Model file for the job. Use its own axes, mm. A direction names the side the tool comes from. Round coordinates to 2 decimals unless told otherwise and drop trailing zeros. Loops run counter-clockwise (first coordinate to the right, second up) from the corner with the lowest first, then second, coordinate; pieces in that order, holes last. Notation, with made-up numbers: M 31,72 L 70,72 A25 ccw 70,104 Z; hole C -38.5,13.5 d10. An arc over 180 degrees is marked long. Use a Markdown table: item, result. Add a question column.
Q1. Cut at B-B (x = 49). Give the cut face in (y, z), plus the area to 3 significant figures.
Q2. Pin check, flat tips, straight feed: pin 1 (0.5 mm diameter, centred on y = 3, z = 1.5, fed in from -X); pin 2 (0.6 mm diameter, centred on x = 28, z = 1, fed in from -Y); pin 3 (1.5 mm diameter, centred on x = 37.5, z = 1.5, fed in from -Y). Stop position of each tip, or through.
Q3. Probe line 1 (X direction, y = 0.75, z = 0.9); line 2 (X direction, y = -1.5, z = 0.6); line 3 (X direction, y = -3, z = 1.1). List the from-to ranges inside material, lowest first. Write a range as from..to.
Q4. Tool access for faces 1 (the face through (9, -4, 3)), 2 (the face through (54.999, -10, 2)), 3 (the face through (16, -2.907, 2)): list every direction of +Z, -Z, +X, -X, +Y, -Y with a clear straight run to the whole face (end or side of a thin tool).
Q5. Cut at D-D (z = 1.25). State how many separate pieces and enclosed holes the cut face has, plus the area to 3 significant figures.
Q6. Cut at C-C (y = 5). Give the cut face in (x, z), plus the area to 3 significant figures.
Q7. Cut at A-A (y = 10.25). Give the cut face in (x, z).
Q8. Mould opens along Y. For faces 4 (the face through (0, -5, 2)), 5 (the face through (47, -8.416, 2)), 6 (the face through (36, -4.416, 2)) say: +Y half, -Y half, draft (parallel to the pull), parting line (faces both ways), or undercut.
from build123d import *

# Parameters (mm, degrees)
SKETCH_1_W          = 2.3276
SKETCH_1_H          = 1.694
EXTRUDE_1_DEPTH     = 3
CUT_EXTRUDE_1_DEPTH = 1


with BuildPart() as part:
    # 草图1 → 凸台-拉伸1 (new body)
    with BuildSketch(Plane.XY.offset(3)):
        with BuildLine():
            Line((23.2531, 5.583631793), (24.503, 5.583631793))
            Line((24.503, 5.583631793), (24.503, 9.583631793))
            Line((24.503, 9.583631793), (18.3721, 9.583631793))
            Line((18.3721, 9.583631793), (18.3721, 12.583631793))
            Line((18.3721, 12.583631793), (12.9991, 12.583631793))
            Line((12.9991, 12.583631793), (12.9991, 7.316491962))
            ThreePointArc((12.9991, 7.316491962), (11.277392164, 3.159921553), (7.120821755, 1.438213717))
            Line((7.120821755, 1.438213717), (0, 1.438213717))
            Line((0, 1.438213717), (0, -11.416368207))
            Line((0, -11.416368207), (7.4994, -11.416368207))
            Line((7.4994, -11.416368207), (7.4994, -8.416368207))
            Line((7.4994, -8.416368207), (36.5002, -8.416368207))
            Line((36.5002, -8.416368207), (36.5002, -4.416368207))
            Line((36.5002, -4.416368207), (35.2489, -4.416368207))
            Line((35.2489, -4.416368207), (35.2489, -1.916368207))
            Line((35.2489, -1.916368207), (36.5002, -1.916368207))
            Line((36.5002, -1.916368207), (36.5002, 1.583631793))
            Line((36.5002, 1.583631793), (39.5003, 1.583631793))
            Line((39.5003, 1.583631793), (39.5003, -1.916368207))
            Line((39.5003, -1.916368207), (40.7501, -1.916368207))
            Line((40.7501, -1.916368207), (40.7501, -4.416368207))
            Line((40.7501, -4.416368207), (39.5003, -4.416368207))
            Line((39.5003, -4.416368207), (39.5003, -8.416368207))
            Line((39.5003, -8.416368207), (54.9988, -8.416368207))
            Line((54.9988, -8.416368207), (54.9988, -11.416368207))
            Line((54.9988, -11.416368207), (59.9998, -11.416368207))
            Line((59.9998, -11.416368207), (59.9998, 12.583631793))
            Line((59.9998, 12.583631793), (51.9988, 12.583631793))
            Line((51.9988, 12.583631793), (51.9988, 9.583631793))
            Line((51.9988, 9.583631793), (27.5031, 9.583631793))
            Line((27.5031, 9.583631793), (27.5031, 5.583631793))
            Line((27.5031, 5.583631793), (28.7543, 5.583631793))
            Line((28.7543, 5.583631793), (28.7543, 3.083631793))
            Line((28.7543, 3.083631793), (27.5031, 3.083631793))
            Line((27.5031, 3.083631793), (27.5031, -0.416368207))
            Line((27.5031, -0.416368207), (24.503, -0.416368207))
            Line((24.503, -0.416368207), (24.503, 3.083631793))
            Line((24.503, 3.083631793), (23.2531, 3.083631793))
            Line((23.2531, 3.083631793), (23.2531, 5.583631793))
        make_face()
        with BuildLine():
            Line((46.2504, 6.082631793), (54.9998, 6.082631793))
            ThreePointArc((54.9998, 6.082631793), (56.414013562, 5.496845355), (56.9998, 4.082631793))
            Line((56.9998, 4.082631793), (56.9998, -2.916368207))
            ThreePointArc((56.9998, -2.916368207), (56.414013562, -4.330581769), (54.9998, -4.916368207))
            Line((54.9998, -4.916368207), (46.2504, -4.916368207))
            ThreePointArc((46.2504, -4.916368207), (44.836186438, -4.330581769), (44.2504, -2.916368207))
            Line((44.2504, -2.916368207), (44.2504, 4.082631793))
            ThreePointArc((44.2504, 4.082631793), (44.836186438, 5.496845355), (46.2504, 6.082631793))
        make_face(mode=Mode.SUBTRACT)
        with Locations((15.811, 3.177631793)):
            Rectangle(SKETCH_1_W, SKETCH_1_H, mode=Mode.SUBTRACT)
        with Locations((15.7586, -2.060368207)):
            Rectangle(SKETCH_1_W, SKETCH_1_H, mode=Mode.SUBTRACT)
    extrude(amount=-EXTRUDE_1_DEPTH)

    # 草图2 → 切除-拉伸1 (cut)
    # profile 1 of 2: a face of its own
    with BuildSketch(Plane.XY.offset(3)):
        Polygon((5.418488838, -1.146310398), (6.065624255, -1.146310398), (6.065624255, -4.646310398), (5.75152169, -4.646310398), (5.75152169, -1.505284757), (5.213060152, -1.505284757), align=None)
    # profile 2 of 2: a face of its own
    with BuildSketch(Plane.XY.offset(3)):
        with BuildLine():
            Line((8.982290921, -1.056566809), (9.22417794, -1.246570815))
            Line((9.22417794, -1.246570815), (8.299398293, -2.660733475))
            add(Edge.make_bspline(
                [(8.299398293, -2.660733475), (8.36096857, -2.650919615), (8.481068357, -2.63177657), (8.602634255, -2.628618624), (8.661878261, -2.627079629)],
                knots=[0, 0, 0, 0, 1.025318673, 2, 2, 2, 2], degree=3))
            add(Edge.make_bspline(
                [(8.661878261, -2.627079629), (8.697450757, -2.628035741), (8.767474158, -2.629917818), (8.87028096, -2.644401669), (8.969069896, -2.667226781), (9.063431508, -2.700499037), (9.15370449, -2.743001391), (9.240406886, -2.793940261), (9.321908896, -2.855945942), (9.399260075, -2.925210897), (9.469487173, -3.001927882), (9.531663228, -3.083329219), (9.58389002, -3.1693301), (9.626263942, -3.259886966), (9.65916882, -3.354860225), (9.683156465, -3.454128365), (9.697336058, -3.557759836), (9.699261549, -3.628238011), (9.700239639, -3.664038764)],
                knots=[0, 0, 0, 0, 1.04369286, 2.054478336, 3.041073146, 4.015093852, 4.984733326, 5.965804835, 6.960378782, 7.985147595, 9.009457201, 10.008161701, 10.986880575, 11.956520048, 12.937015923, 13.931873656, 14.949455224, 16, 16, 16, 16], degree=3))
            add(Edge.make_bspline(
                [(9.700239639, -3.664038764), (9.698816534, -3.713018468), (9.696016201, -3.809398934), (9.668112405, -3.94977564), (9.62475276, -4.083508155), (9.562775231, -4.208461327), (9.485792849, -4.324463896), (9.391915256, -4.427249362), (9.284471767, -4.518919399), (9.162984969, -4.595576018), (9.032242005, -4.658179069), (8.894890008, -4.703144311), (8.752262861, -4.730827781), (8.655458253, -4.734298384), (8.606489639, -4.736053988)],
                knots=[0, 0, 0, 0, 1.031375318, 2.029502543, 3.004789286, 3.987476834, 4.960371455, 5.9300674, 6.912260825, 7.929083631, 8.949397511, 9.960523116, 10.96833055, 12, 12, 12, 12], degree=3))
            add(Edge.make_bspline(
                [(8.606489639, -4.736053988), (8.559392939, -4.734525782), (8.466102621, -4.731498674), (8.328869826, -4.704532736), (8.197006809, -4.660825634), (8.071437428, -4.600611355), (7.955116815, -4.524553472), (7.851051179, -4.432991193), (7.759759404, -4.327881728), (7.683784783, -4.209241381), (7.623526051, -4.081751423), (7.578336126, -3.948814267), (7.551939883, -3.810914285), (7.548251326, -3.717433146), (7.546393485, -3.67034886)],
                knots=[0, 0, 0, 0, 1.012016664, 2.004627821, 2.994792927, 3.992885782, 4.990978636, 5.973936114, 6.964471063, 7.975201453, 8.993600317, 9.990122807, 10.98767138, 12, 12, 12, 12], degree=3))
            add(Edge.make_bspline(
                [(7.546393485, -3.67034886), (7.54757493, -3.634304277), (7.549987215, -3.560708125), (7.566830606, -3.449244097), (7.5938954, -3.335193015), (7.624205647, -3.238438821), (7.656231257, -3.159177299), (7.682883796, -3.095273809), (7.716057792, -3.029512736), (7.751431174, -2.9596391), (7.792188043, -2.887453667), (7.836503692, -2.811749997), (7.885603343, -2.73373207), (7.920023506, -2.680787874), (7.937619447, -2.653722257)],
                knots=[0, 0, 0, 0, 1.173818275, 2.396712641, 3.66331629, 4.989737886, 5.693666774, 6.447286557, 7.243889047, 8.091586357, 8.998013824, 9.943181721, 10.948533338, 12, 12, 12, 12], degree=3))
            Line((7.937619447, -2.653722257), (8.982290921, -1.056566809))
        make_face()
        with BuildLine():
            add(Edge.make_bspline(
                [(8.595972812, -2.986053988), (8.569310567, -2.986832032), (8.517231458, -2.988351777), (8.440824043, -2.997177029), (8.368510792, -3.013796095), (8.299333658, -3.034962426), (8.234585955, -3.064065486), (8.173797115, -3.099417285), (8.116732064, -3.141038463), (8.063988512, -3.188339374), (8.016168848, -3.240127407), (7.974987718, -3.29559693), (7.939465318, -3.353411133), (7.910583499, -3.414053075), (7.888093423, -3.477499574), (7.871825172, -3.543458824), (7.862771421, -3.61237313), (7.861265189, -3.659105633), (7.860496049, -3.682969052)],
                knots=[0, 0, 0, 0, 1.129588631, 2.206414736, 3.251139165, 4.268635594, 5.265702196, 6.250456724, 7.242448911, 8.251968645, 9.246821453, 10.222880186, 11.173611482, 12.116736599, 13.062300278, 14.020270554, 14.989073742, 16, 16, 16, 16], degree=3))
            add(Edge.make_bspline(
                [(7.860496049, -3.682969052), (7.861122411, -3.706619032), (7.862350613, -3.752993122), (7.873502932, -3.821332301), (7.890538015, -3.88709721), (7.915878411, -3.949948808), (7.946105299, -4.010845127), (7.986010623, -4.067580412), (8.030227409, -4.123600482), (8.083081342, -4.174601954), (8.139804705, -4.222058578), (8.200405908, -4.263538831), (8.263565868, -4.299025005), (8.33013729, -4.326836102), (8.399175674, -4.349660389), (8.471256228, -4.365721868), (8.546429083, -4.374802394), (8.597351021, -4.376310588), (8.623316562, -4.377079629)],
                knots=[0, 0, 0, 0, 0.989467248, 1.94019797, 2.891935182, 3.827694429, 4.772920941, 5.730924762, 6.725747692, 7.756678648, 8.79901574, 9.819492441, 10.826891316, 11.826466727, 12.835195252, 13.867842842, 14.912794438, 16, 16, 16, 16], degree=3))
            add(Edge.make_bspline(
                [(8.623316562, -4.377079629), (8.649282061, -4.376310528), (8.700203915, -4.374802216), (8.775377376, -4.365722547), (8.847455694, -4.349657899), (8.916502203, -4.326845129), (8.983043634, -4.298991519), (9.046148355, -4.263759599), (9.106176449, -4.221803482), (9.162937048, -4.174683053), (9.215570987, -4.123310201), (9.260848266, -4.068080479), (9.299531499, -4.010386584), (9.330965686, -3.950188694), (9.356026977, -3.887059206), (9.373148445, -3.821342482), (9.384277733, -3.752990456), (9.3855091, -3.706618132), (9.386137075, -3.682969052)],
                knots=[0, 0, 0, 0, 1.087397944, 2.132534446, 3.165364764, 4.174271784, 5.174024072, 6.181601208, 7.194203697, 8.236725232, 9.267838612, 10.269026844, 11.221737037, 12.171628256, 13.107553087, 14.05945871, 15.010357665, 16, 16, 16, 16], degree=3))
            add(Edge.make_bspline(
                [(9.386137075, -3.682969052), (9.385586782, -3.659074501), (9.384506736, -3.612177269), (9.372290787, -3.54348965), (9.355348413, -3.477164444), (9.329765383, -3.413618495), (9.296528838, -3.353102568), (9.256045431, -3.295310967), (9.209212861, -3.23980062), (9.155115321, -3.188237811), (9.096225087, -3.141090733), (9.033609502, -3.099471177), (8.968101528, -3.0643462), (8.899767586, -3.035039098), (8.827824703, -3.013889624), (8.753434364, -2.997236381), (8.675645121, -2.988374363), (8.622868513, -2.986837298), (8.595972812, -2.986053988)],
                knots=[0, 0, 0, 0, 0.978206639, 1.919901502, 2.851605144, 3.780102724, 4.718870031, 5.675451981, 6.667674623, 7.690630536, 8.733308323, 9.756129687, 10.767539656, 11.776269907, 12.797430371, 13.836405707, 14.897401972, 16, 16, 16, 16], degree=3))
        make_face(mode=Mode.SUBTRACT)
    extrude(amount=-CUT_EXTRUDE_1_DEPTH, mode=Mode.SUBTRACT)


solid = part.part
Checked values:
| question | item | result |
|---|---|---|
| 1 | outline | M -8.42,0 L -4.92,0 L -4.92,3 L -8.42,3 Z; M 6.08,0 L 9.58,0 L 9.58,3 L 6.08,3 Z |
| 1 | area | 21.0 mm^2 |
| 2 | pin 1 | stops at x = 10.82 |
| 2 | pin 2 | stops at y = -8.42 |
| 2 | pin 3 | stops at y = 1.58 |
| 3 | line 1 | x = 0..24.5, 27.5..36.5, 39.5..44.25, 57..60 |
| 3 | line 2 | x = 0..14.59, 16.92..36.5, 39.5..44.25, 57..60 |
| 3 | line 3 | x = 0..35.25, 40.75..44.25, 57..60 |
| 4 | face 1 | +Z, +X, -X, +Y, -Y |
| 4 | face 2 | +Z, -Z, -Y |
| 4 | face 3 | +Z, -Z |
| 5 | separate pieces | 1 |
| 5 | enclosed holes | 3 |
| 5 | area | 842 mm^2 |
| 6 | outline | M 12.52,0 L 23.25,0 L 23.25,3 L 12.52,3 Z; M 28.75,0 L 44.47,0 L 44.47,3 L 28.75,3 Z; M 56.78,0 L 60,0 L 60,3 L 56.78,3 Z |
| 6 | area | 89.0 mm^2 |
| 7 | outline | M 13,0 L 18.37,0 L 18.37,3 L 13,3 Z; M 52,0 L 60,0 L 60,3 L 52,3 Z |
| 8 | face 4 | draft |
| 8 | face 5 | -Y half |
| 8 | face 6 | undercut |
